from build123d import *

# Parameters (mm, degrees)
SKETCH1_W                = 381
SKETCH1_H                = 406.4
BOSS_EXTRUDE1_DEPTH      = 12.7
CUT_EXTRUDE1_DEPTH       = 530.86
BOSS_EXTRUDE2_DEPTH      = 190.5
BOSS_EXTRUDE2_DEPTH_BACK = 190.5
CUT_EXTRUDE2_DEPTH       = 185.42
CUT_EXTRUDE2_DEPTH_BACK  = 185.42
SKETCH9_W                = 370.84
SKETCH9_H                = 38.1
BOSS_EXTRUDE3_DEPTH      = 203.2
SKETCH9_2_W              = 370.84
SKETCH9_2_H              = 38.1
CUT_EXTRUDE3_DEPTH       = 200.66
FILLET12_R               = 2.54
SKETCH20_W               = 381
SKETCH20_H               = 12.7
BOSS_EXTRUDE5_DEPTH      = 406.4
CUT_EXTRUDE10_DEPTH      = 304.8
CUT_EXTRUDE10_DEPTH_BACK = 259.334
SKETCH27_W               = 25.4
SKETCH27_H               = 12.7
SKETCH27_R               = 3.175
BOSS_EXTRUDE6_DEPTH      = 184.15
BOSS_EXTRUDE6_DEPTH_BACK = 184.15
SKETCH27_2_W             = 25.4
SKETCH27_2_H             = 12.7
SKETCH27_2_R             = 3.175
CUT_EXTRUDE11_DEPTH      = 177.8
CUT_EXTRUDE11_DEPTH_BACK = 177.8
FILLET14_R               = 5.08
SKETCH29_W               = 6.35
SKETCH29_H               = 38.1
CUT_EXTRUDE12_DEPTH      = 229.6
CUT_EXTRUDE12_DEPTH_BACK = 204.2000001


with BuildPart() as part:
    # Sketch1 → Boss-Extrude1 (new body)
    with BuildSketch(Plane(origin=(0, 0, 0), x_dir=(1, 0, 0), z_dir=(0, 1, 0))):
        Rectangle(SKETCH1_W, SKETCH1_H)
    extrude(amount=-BOSS_EXTRUDE1_DEPTH)

    # Sketch5 → Cut-Extrude1 (cut)
    with BuildSketch(Plane(origin=(0, 0, -203.2), x_dir=(-1, 0, 0), z_dir=(0, 0, -1))):
        Polygon((190.5, 0), (0, -12.7), (190.5, -12.7), align=None)
        Polygon((0, -12.7), (-190.5, 0), (-190.5, -12.7), align=None)
    extrude(amount=-CUT_EXTRUDE1_DEPTH, mode=Mode.SUBTRACT)

    # Sketch6 → Boss-Extrude2 (add, two sides)
    with BuildSketch(Plane(origin=(0, 0, 0), x_dir=(0, 0, -1), z_dir=(1, 0, 0))) as boss_extrude2_sk:
        with BuildLine():
            Line((-203.2, 0), (-203.2, 38.1))
            add(Edge.make_bspline(
                [(-203.2, 38.1), (-139.671233151, 43.854392756), (-4.575804842, 44.131584557), (127.011271564, 22.260123732), (203.2, 0)],
                knots=[0, 0, 0, 0, 0.446112954, 1, 1, 1, 1], degree=3))
            Line((203.2, 0), (-203.2, 0))
        make_face()
    extrude(amount=BOSS_EXTRUDE2_DEPTH)
    extrude(boss_extrude2_sk.sketch, amount=-BOSS_EXTRUDE2_DEPTH_BACK)

    # Sketch6<2> → Cut-Extrude2 (cut, two sides)
    with BuildSketch(Plane(origin=(0, 0, 0), x_dir=(0, 0, -1), z_dir=(1, 0, 0))) as cut_extrude2_sk:
        with BuildLine():
            Line((-203.2, 0), (-203.2, 38.1))
            add(Edge.make_bspline(
                [(-203.2, 38.1), (-139.671233151, 43.854392756), (-4.575804842, 44.131584557), (127.011271564, 22.260123732), (203.2, 0)],
                knots=[0, 0, 0, 0, 0.446112954, 1, 1, 1, 1], degree=3))
            Line((203.2, 0), (-203.2, 0))
        make_face()
    extrude(amount=CUT_EXTRUDE2_DEPTH, mode=Mode.SUBTRACT)
    extrude(cut_extrude2_sk.sketch, amount=-CUT_EXTRUDE2_DEPTH_BACK, mode=Mode.SUBTRACT)

    # Sketch9 → Boss-Extrude3 (add)
    with BuildSketch(Plane.XY):
        with Locations((0, 19.05)):
            Rectangle(SKETCH9_W, SKETCH9_H)
    extrude(amount=BOSS_EXTRUDE3_DEPTH)

    # Sketch9<2> → Cut-Extrude3 (cut)
    with BuildSketch(Plane.XY):
        with Locations((0, 19.05)):
            Rectangle(SKETCH9_2_W, SKETCH9_2_H)
    extrude(amount=CUT_EXTRUDE3_DEPTH, mode=Mode.SUBTRACT)

    # Fillet12
    fillet12_edges = [part.edges().sort_by_distance(p)[0] for p in [
        (0, 0, 200.66),
    ]]
    fillet(fillet12_edges, radius=FILLET12_R)

    # Sketch20 → Boss-Extrude5 (add)
    with BuildSketch(Plane.XY.offset(203.2)):
        with Locations((0, -6.35)):
            Rectangle(SKETCH20_W, SKETCH20_H)
    extrude(amount=-BOSS_EXTRUDE5_DEPTH)

    # Sketch21 → Cut-Extrude10 (cut, two sides)
    with BuildSketch(Plane(origin=(0, 0, 0), x_dir=(0, 0, -1), z_dir=(1, 0, 0))) as cut_extrude10_sk:
        with BuildLine():
            Line((-203.2, 38.1), (-203.2, 89.275464314))
            Line((-203.2, 89.275464314), (140.49634993, 63.687732157))
            Line((140.49634993, 63.687732157), (140.49634993, 16.247140788))
            add(Edge.make_bspline(
                [(-203.2, 38.1), (-32.059595942, 17.691928411), (140.49634993, 16.247140788)],
                knots=[0, 0, 0, 1, 1, 1], degree=2))
        make_face()
    extrude(amount=CUT_EXTRUDE10_DEPTH, mode=Mode.SUBTRACT)
    extrude(cut_extrude10_sk.sketch, amount=-CUT_EXTRUDE10_DEPTH_BACK, mode=Mode.SUBTRACT)

    # Sketch27 → Boss-Extrude6 (add, two sides)
    with BuildSketch(Plane(origin=(0, 0, 0), x_dir=(0, 0, -1), z_dir=(1, 0, 0))) as boss_extrude6_sk:
        with Locations((-215.9, 29.21)):
            Rectangle(SKETCH27_W, SKETCH27_H)
        with Locations((-222.25, 29.21)):
            Circle(SKETCH27_R, mode=Mode.SUBTRACT)
    extrude(amount=BOSS_EXTRUDE6_DEPTH)
    extrude(boss_extrude6_sk.sketch, amount=-BOSS_EXTRUDE6_DEPTH_BACK)

    # Sketch27<2> → Cut-Extrude11 (cut, two sides)
    with BuildSketch(Plane(origin=(0, 0, 0), x_dir=(0, 0, -1), z_dir=(1, 0, 0))) as cut_extrude11_sk:
        with Locations((-215.9, 29.21)):
            Rectangle(SKETCH27_2_W, SKETCH27_2_H)
        with Locations((-222.25, 29.21)):
            Circle(SKETCH27_2_R, mode=Mode.SUBTRACT)
    extrude(amount=CUT_EXTRUDE11_DEPTH, mode=Mode.SUBTRACT)
    extrude(cut_extrude11_sk.sketch, amount=-CUT_EXTRUDE11_DEPTH_BACK, mode=Mode.SUBTRACT)

    # Fillet14
    fillet14_edges = [part.edges().sort_by_distance(p)[0] for p in [
        (-180.975, 22.86, 228.6),
        (-180.975, 35.56, 228.6),
        (180.975, 35.56, 228.6),
        (180.975, 22.86, 228.6),
    ]]
    fillet(fillet14_edges, radius=FILLET14_R)

    # Sketch29 → Cut-Extrude12 (cut, two sides)
    with BuildSketch(Plane.XY) as cut_extrude12_sk:
        with Locations((-187.325, 19.05)):
            Rectangle(SKETCH29_W, SKETCH29_H)
        with Locations((187.325, 19.05)):
            Rectangle(SKETCH29_W, SKETCH29_H)
    extrude(amount=CUT_EXTRUDE12_DEPTH, mode=Mode.SUBTRACT)
    extrude(cut_extrude12_sk.sketch, amount=-CUT_EXTRUDE12_DEPTH_BACK, mode=Mode.SUBTRACT)


solid = part.part
Input: part model. Units: mm. Frame: model coordinates. A direction names the side the tool comes from. Give positions to 0.01 mm unless a question says otherwise; leave off trailing zeros. Loops run counter-clockwise (first coordinate to the right, second up) from the corner with the lowest first, then second, coordinate; pieces in that order, holes last. Notation, with made-up numbers: M -31.75,59 L 11.25,59 A30 cw 11.25,87 Z; hole C -15,-2 d3. An arc over 180 degrees is marked long. Use CSV: the item, a comma, the result in double quotes.
(1) Set-up query: faces 1 (the face through (-184.15, 28, 212)), 2 (the face through (177.8, 29, 216)), 3 (the face through (190.5, -6, 3)), 4 (the face through (-3, 20, 200.66)), 5 (the face through (184.15, 26, 212)). Return all of +Z, -Z, +X, -X, +Y, -Y with unobstructed straight access to the full face (end or side cutting, diameter ignored); none if empty.
Outcome:
face 1,"+Z, -Z, -X, +Y"
face 2,"+Z, +Y, -Y"
face 3,"+Z, -Z, +X, +Y, -Y"
face 4,"-Z, +X, -X, +Y"
face 5,"+Z, -Z, +X, +Y"
(2) Pin query (flat end, axial travel): P1, Ø24.5, axis at y = 11.5, z = 216, coming from the +X side; P2, Ø1.5, axis at x = 38, y = 5.5, coming from the +Z side; P3, Ø7, axis at x = -182, z = 214.5, coming from the -Y side. Return the tip coordinate at first contact, or that it passes through.
Outcome:
P1,"stops at x = 184.15"
P2,"stops at z = 203.2"
P3,"stops at y = 22.86"
(3) Section B-B, the plane y = -6. Return loops of the section in (x, z), plus the area to 3 significant figures.
Outcome:
outline,"M -190.5,-203.2 L 190.5,-203.2 L 190.5,203.2 L -190.5,203.2 Z"
area,"155,000 mm²"
(4) Section A-A, the plane z = -91.5. Return loops of the section in (x, y), plus the area to 3 significant figures.
Outcome:
outline,"M -190.5,-12.7 L 190.5,-12.7 L 190.5,0 L -190.5,0 Z"
area,"4,840 mm²"
(5) Material intervals for L1, parallel to Y at x = -181.5, z = 222.25 (3 decimals); L2, parallel to Z at x = -181, y = 29; L3, parallel to Y at x = 12.5, z = -57, sorted ascending. Write a range as [from, to].
Outcome:
L1,"y = [22.86, 26.035], [32.385, 35.56]"
L2,"z = [200.66, 219.08], [225.42, 228.6]"
L3,"y = [-12.7, 0]"
(6) Pull-direction query (X, two-part tool) for faces 6 (the face through (-190.5, -6, 3)), 7 (the face through (-3, -12.7, 3)), 8 (the face through (-3, 13, 203.2)); classes: pulls with the +X half, pulls with the -X half, needs draft (parallel to the pull), parting line crosses it, or undercut.
Outcome:
face 6,"pulls with the -X half"
face 7,"needs draft"
face 8,"undercut"
